from build123d import *

# Parameters (mm, degrees)
BOSS_EXTRUDE1_DEPTH     = 5
CUT_EXTRUDE4_DEPTH      = 271.785893281
CUT_EXTRUDE4_DEPTH_BACK = 271.785893281
SKETCH3_R               = 7.5
CUT_EXTRUDE5_DEPTH      = 271.785893281
CUT_EXTRUDE5_DEPTH_BACK = 271.785893281
SKETCH5_R               = 7.5


with BuildPart() as part:
    # Sketch1 → Boss-Extrude1 (new body)
    with BuildSketch(Plane.XY):
        with BuildLine():
            Line((-20, 0), (-20, 250))
            ThreePointArc((-20, 250), (0, 270), (20, 250))
            Line((20, 250), (20, 0))
            ThreePointArc((20, 0), (0, -20), (-20, 0))
        make_face()
    extrude(amount=BOSS_EXTRUDE1_DEPTH)

    # Sketch3 → Cut-Extrude4 (cut, two sides: drawn at the far end of the back side and taken through both)
    with BuildSketch(Plane.XY.offset(-CUT_EXTRUDE4_DEPTH_BACK)):
        with Locations((0, 260)):
            Circle(SKETCH3_R)
        with Locations((0, -10)):
            Circle(SKETCH3_R)
    extrude(amount=CUT_EXTRUDE4_DEPTH + CUT_EXTRUDE4_DEPTH_BACK, mode=Mode.SUBTRACT)

    # Sketch5 → Cut-Extrude5 (cut, two sides: drawn at the far end of the back side and taken through both)
    with BuildSketch(Plane.XY.offset(5).offset(-CUT_EXTRUDE5_DEPTH_BACK)):
        with Locations((0, 129.974184192)):
            Circle(SKETCH5_R)
    extrude(amount=CUT_EXTRUDE5_DEPTH + CUT_EXTRUDE5_DEPTH_BACK, mode=Mode.SUBTRACT)


solid = part.part
Geometry: final body of the model. Coordinates: model frame, mm. Coordinates: 2 decimals unless noted, no trailing zeros. Order: outer loops, then holes, each group sorted by start corner. A loop starts at its lowest first (then second) coordinate and runs counter-clockwise, first axis right, second up.
(1) Section query B-B (z = 3.2). Return the cut outline in (x, y).
(2) Section query C-C (y = -10). Return the cut outline in (x, z).
(3) Material intervals for probe 1 along Y at (x, z) = (0, 1.65); probe 2 along Y at (x, z) = (-4.5, 1.05); probe 3 along X at (y, z) = (-10, 2.5), sorted ascending.
(4) Section query D-D (x = -14). Return the cut outline in (y, z).
(5) Draft query along Y for faces 1 (the face through (0, -20, 2)), 2 (the face through (-9, 127, 5)), 3 (the face through (6.928, 127.102, 2.465)). Return one class per face: pulls with the +Y half, pulls with the -Y half, needs draft (parallel to the pull), parting line crosses it, or undercut.
(6) Section query A-A (x = 1). Return the cut outline in (y, z).
(7) First-contact query: pin 1 (2 mm diameter, centred on x = 15, z = 2, fed in from -Y). Flat tip, straight axial feed; report the tip coordinate or a pass-through.
Solution:
1. outline: (-20, 0) arc R20 ccw to (20, 0) - (20, 250) arc R20 ccw to (-20, 250) - close; hole circle Ø15 at (0, -10); hole circle Ø15 at (0, 129.97); hole circle Ø15 at (0, 260)
2. outline: (-17.32, 0) - (-7.5, 0) - (-7.5, 5) - (-17.32, 5) - close; (7.5, 0) - (17.32, 0) - (17.32, 5) - (7.5, 5) - close
3. probe 1: y = -20 to -17.5, -2.5 to 122.47, 137.47 to 252.5, 267.5 to 270
3. probe 2: y = -19.49 to -16, -4 to 123.97, 135.97 to 254, 266 to 269.49
3. probe 3: x = -17.32 to -7.5, 7.5 to 17.32
4. outline: (-14.28, 0) - (264.28, 0) - (264.28, 5) - (-14.28, 5) - close
5. face 1: pulls with the -Y half
5. face 2: needs draft
5. face 3: undercut
6. outline: (-19.97, 0) - (-17.43, 0) - (-17.43, 5) - (-19.97, 5) - close; (-2.57, 0) - (122.54, 0) - (122.54, 5) - (-2.57, 5) - close; (137.41, 0) - (252.57, 0) - (252.57, 5) - (137.41, 5) - close; (267.43, 0) - (269.97, 0) - (269.97, 5) - (267.43, 5) - close
7. pin 1: stops at y = -14.28
